Input: part model. Units: mm. Frame: model coordinates. Face numbers are marked on the shaded views. A direction names the side the tool comes from. Round coordinates to 2 decimals unless told otherwise and drop trailing zeros. Loops run counter-clockwise (first coordinate to the right, second up) from the corner with the lowest first, then second, coordinate; pieces in that order, holes last. Notation, with made-up numbers: (22.5, 41.25) -> (66.5, 41.25) arc R30 ccw to (66.5, 65.25) -> close; hole circle Ø11 at (47, 73). An arc over 180 degrees is marked (long way). Answer in a Markdown table with one row per item. Add a question column.
Q1. Reachability of the marked faces 1 and 2 from +Z, -Z, +X, -X, +Y, -Y: full face, straight path, thin tool, end or side. Return the list, or none.
Q2. Section A-A, the plane x = -7.5. Output: boundary loops of the cut face in (y, z), and give its area (3 significant figures).
Q3. Ray query, L1, parallel to Y at x = 0, z = 3.35; L2, parallel to Y at x = 80, z = 4.55; L3, parallel to X at y = -3, z = 5.75. Return the intervals inside material, ascending. Write a range as from..to.
Q4. Mould query, pull axis Y, two halves, no side actions, for the marked faces 3, 4 and 5. Classes: pulls with the +Y half, pulls with the -Y half, needs draft (parallel to the pull), parting line crosses it, or undercut.
Q5. Section C-C, the plane y = -15.5. Output: boundary loops of the cut face in (x, z), and give its area (3 significant figures).
Q6. Section B-B, the plane z = 3.75. Give the number of separate pieces and of enclosed holes in the cut face, and give its area (3 significant figures).
```python
from build123d import *

# Parameters (mm, degrees)
ESQUISSE1_R             = 18.5
ESQUISSE1_R_2           = 1.1
ESQUISSE1_R_3           = 12.5
BOSS_EXTRU_1_DEPTH      = 6
BOSS_EXTRU_2_START      = -6
ESQUISSE2_R             = 4.5
BOSS_EXTRU_2_DEPTH      = 6
ENL_V_MAT_EXTRU_1_DEPTH = 90.244943834
CONG_1_R                = 6
BOSS_EXTRU_3_START      = -6
ESQUISSE4_R             = 1.5
BOSS_EXTRU_3_DEPTH      = 6


with BuildPart() as part:
    # Esquisse1 → Boss.-Extru.1 (new body)
    with BuildSketch(Plane.XY):
        Circle(ESQUISSE1_R)
        with Locations((0, 15.5)):
            Circle(ESQUISSE1_R_2, mode=Mode.SUBTRACT)
        with Locations((15.5, 0)):
            Circle(ESQUISSE1_R_2, mode=Mode.SUBTRACT)
        with Locations((0, -15.5)):
            Circle(ESQUISSE1_R_2, mode=Mode.SUBTRACT)
        with Locations((-15.5, 0)):
            Circle(ESQUISSE1_R_2, mode=Mode.SUBTRACT)
        Circle(ESQUISSE1_R_3, mode=Mode.SUBTRACT)
    extrude(amount=BOSS_EXTRU_1_DEPTH)

    # Esquisse2 → Boss.-Extru.2 (add)
    with BuildSketch(Plane.XY.offset(6).offset(BOSS_EXTRU_2_START)):
        with BuildLine():
            Line((2.63625, 18.311203836), (81.01175, 7.027543094))
            ThreePointArc((81.01175, 7.027543094), (87.1, 0), (81.01175, -7.027543094))
            Line((81.01175, -7.027543094), (2.63625, -18.311203836))
            ThreePointArc((2.63625, -18.311203836), (18.5, 0), (2.63625, 18.311203836))
        make_face()
        with Locations((80, 0)):
            Circle(ESQUISSE2_R, mode=Mode.SUBTRACT)
    extrude(amount=BOSS_EXTRU_2_DEPTH)

    # Esquisse3 → Enlèv. mat.-Extru.1 (cut, through all)
    with BuildSketch(Plane.XY.offset(6)):
        with BuildLine():
            Line((13.438126494, 12.714824274), (74.119447809, 3.978580893))
            ThreePointArc((74.119447809, 3.978580893), (72.9, 0), (74.119447809, -3.978580893))
            Line((74.119447809, -3.978580893), (13.438126494, -12.714824274))
            ThreePointArc((13.438126494, -12.714824274), (18.5, 0), (13.438126494, 12.714824274))
        make_face()
    extrude(amount=-ENL_V_MAT_EXTRU_1_DEPTH, mode=Mode.SUBTRACT)

    # Congé1
    # the kernel refuses this fillet: 6 mm, written as the material it adds along each edge
    with BuildSketch(Plane(origin=(74.119447809, -3.978580893, 6), x_dir=(-0.989794801966549, -0.1424999999999999, 0), z_dir=(0, 0, -1))) as cong_1_piece_1:
        with BuildLine():
            CenterArc((6.387487769, 6), CONG_1_R, 192.789750134, 77.210249866)
            ThreePointArc((0.536353935, 4.671755725), (0.666177836, 2.290184264), (0, 0))
            Line((0, 0), (6.387487769, 0))
        make_face()
    extrude(amount=6)
    with BuildSketch(Plane(origin=(74.119447809, 3.978580893, 6), x_dir=(-0.25446461339287313, -0.9670820857253097, 0), z_dir=(0, 0, -1))) as cong_1_piece_2:
        with BuildLine():
            CenterArc((6.689391795, 5.661451882), CONG_1_R, 173.450673101, 77.210249866)
            Line((0.728547621, 6.345803209), (0, 0))
            ThreePointArc((0, 0), (2.351221868, 0.400615273), (4.702443737, 0))
        make_face()
    extrude(amount=6)
    with BuildSketch(Plane(origin=(13.438126494, -12.714824274, 6), x_dir=(0.46579561947351233, 0.8848923329305587, 0), z_dir=(0, 0, -1))) as cong_1_piece_3:
        with BuildLine():
            CenterArc((11.602632031, 5.777450125), CONG_1_R, 144.04573826, 110.300190842)
            Line((6.745716297, 9.300285568), (0, 0))
            ThreePointArc((0, 0), (4.99183006, 0.686195447), (9.98366012, 0))
        make_face()
    extrude(amount=6)
    with BuildSketch(Plane(origin=(13.438126494, 12.714824274, 6), x_dir=(0.4657956194735124, -0.8848923329305588, 0), z_dir=(0, 0, -1))) as cong_1_piece_4:
        with BuildLine():
            CenterArc((11.602632031, -5.777450125), CONG_1_R, 105.654070898, 110.300190842)
            Line((6.745716297, -9.300285568), (0, 0))
            ThreePointArc((0, 0), (4.99183006, -0.686195447), (9.98366012, 0))
        make_face()
    extrude(amount=6)

    # Esquisse4 → Boss.-Extru.3 (add)
    with BuildSketch(Plane.XY.offset(6).offset(BOSS_EXTRU_3_START)):
        with BuildLine():
            Line((82.706875, 6.563751041), (96.38125, 0.924471978))
            ThreePointArc((96.38125, 0.924471978), (97, 0), (96.38125, -0.924471978))
            Line((96.38125, -0.924471978), (82.706875, -6.563751041))
            ThreePointArc((82.706875, -6.563751041), (87.1, 0), (82.706875, 6.563751041))
        make_face()
        with Locations((90, 0)):
            Circle(ESQUISSE4_R, mode=Mode.SUBTRACT)
    extrude(amount=BOSS_EXTRU_3_DEPTH)


solid = part.part
```
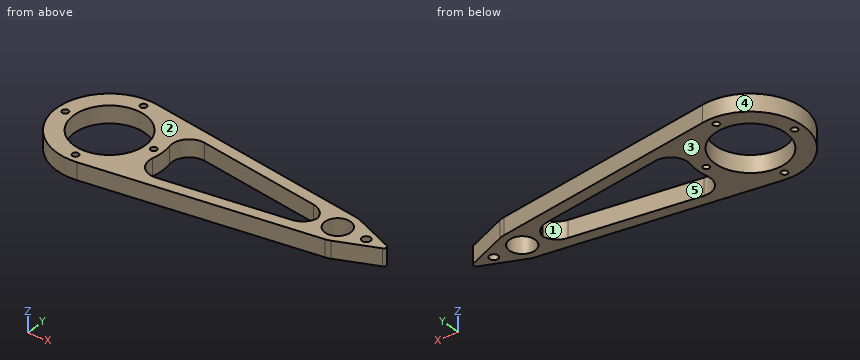
Answer block:
| question | item | result |
|---|---|---|
| 1 | face 1 | +Z, -Z |
| 1 | face 2 | +Z, +X, -X, +Y, -Y |
| 2 | outline | (-16.91, 0) -> (-10, 0) -> (-10, 6) -> (-16.91, 6) -> close; (10, 0) -> (16.91, 0) -> (16.91, 6) -> (10, 6) -> close |
| 2 | area | 82.9 mm^2 |
| 3 | L1 | -18.5..-16.6, -14.4..-12.5, 12.5..14.4, 16.6..18.5 |
| 3 | L2 | -7.17..-4.5, 4.5..7.17 |
| 3 | L3 | -18.26..-12.13, 12.13..18.26, 71.37..76.65, 83.35..91.35 |
| 4 | face 3 | needs draft |
| 4 | face 4 | parting line crosses it |
| 4 | face 5 | undercut |
| 5 | outline | (-10.1, 0) -> (-1.1, 0) -> (-1.1, 6) -> (-10.1, 6) -> close; (1.1, 0) -> (22.16, 0) -> (22.16, 6) -> (1.1, 6) -> close |
| 5 | area | 180 mm^2 |
| 6 | separate pieces | 1 |
| 6 | enclosed holes | 8 |
| 6 | area | 1,310 mm^2 |
